```python
from build123d import *

# Parameters (mm, degrees)
F2_R = 25.4
F3_T = -1.27


with BuildPart() as f1:
    # F0 (on Front) → F1 (revolve)
    with BuildSketch(Plane.XZ):
        Polygon((-36.2194851041, -76.4004662633), (0, -76.4004662633), (0, 50.3677166998), (-35.8421988785, 50.3677166998), (-35.8421988785, 6.2252227217), (-4.1501536034, -8.8662281632), (-4.1501536034, -71.1184665561), align=None)
    revolve(axis=Axis((0, 0, -13.0163747817), (0, 0, -1)))

    # F2
    f2_edges = [f1.edges().sort_by_distance(p)[0] for p in [
        (35.842199, 0, 6.225223),
    ]]
    fillet(f2_edges, radius=F2_R)

    # F3
    f3_openings = [f1.faces().sort_by_distance(p)[0] for p in [
        (0, 0, 50.367717),
    ]]
    offset(amount=F3_T, openings=f3_openings, kind=Kind.INTERSECTION)


solid = f1.part
```
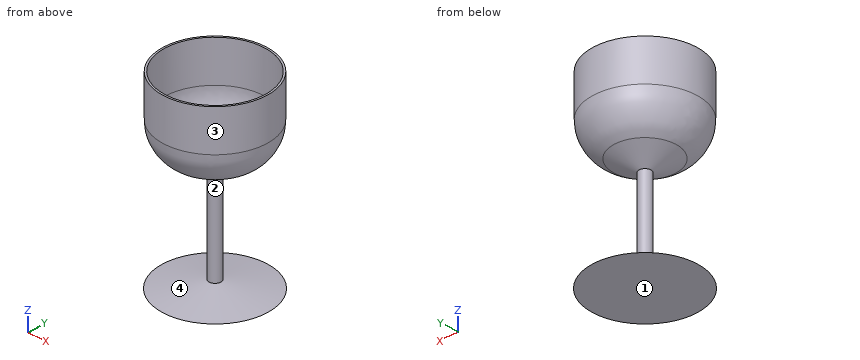
Could you check a few things on this model? Use its own coordinates, in mm. Face numbers are marked on the shaded views. A direction names the side the tool comes from. Coordinates: 2 decimals unless noted, no trailing zeros. Order: outer loops, then holes, each group sorted by start corner. A loop starts at its lowest first (then second) coordinate and runs counter-clockwise, first axis right, second up. Notation, with made-up numbers: M 79.5,65 L 128.5,65 A22 ccw 128.5,99 Z; hole C -4.5,85 d11. An arc over 180 degrees is marked long. Use one line per item in the form item = value. Start each with the question number.
1. On a 3-axis mill with a long thin cutter (end or side, diameter ignored), from which of +Z, -Z, +X, -X, +Y, -Y can I reach the whole of each face in a straight line? I mean the marked faces 3 and 4. Say none if no direction works.
2. We'd pull the mould along Z, two halves only. Please class the marked faces 1 and 2: +Z half, -Z half, draft (parallel to the pull), parting line (faces both ways), or undercut.
3. Please list where these lines run through material, in increasing order: line 1 (Z direction, x = -6, y = 10.5); line 2 (Z direction, x = -6, y = 12.5); line 3 (Y direction, x = 0, z = -37).
4. Suppose I cut it at A-A on x = 11.5. Count the separate pieces of the cut face and the enclosed holes in it, then the cut area to 3 significant figures.
5. For pin 1 (6 mm diameter, centred on x = 14.5, z = 33, fed in from +Y); pin 2 (1.5 mm diameter, centred on y = -21, z = 32.5, fed in from -X); pin 3 (2 mm diameter, centred on x = -4.5, z = -39, fed in from -Y), each with a flat end and sliding along its axis, tell me the tip position at first contact or that it passes through.
6. Suppose I cut it at C-C on z = -12.5. Write out the boundary of the cut face in (x, y).
Geometry says:
q1.face_3 = +Z
q1.face_4 = none
q2.face_1 = -Z half
q2.face_2 = undercut
q3.line_1 = -76.4 to -75.13, -73.71 to -72.43, -5.08 to -3.68
q3.line_2 = -76.4 to -75.13, -74.01 to -72.72, -4.24 to -2.83
q3.line_3 = -4.15 to -2.88, 2.88 to 4.15
q4.separate_pieces = 2
q4.enclosed_holes = 1
q4.area = 335 mm^2
q5.pin_1 = 33.95
q5.pin_2 = -29.57
q5.pin_3 = -2.23
q6.outline = C 0,0 d8.3; hole C 0,0 d5.76
